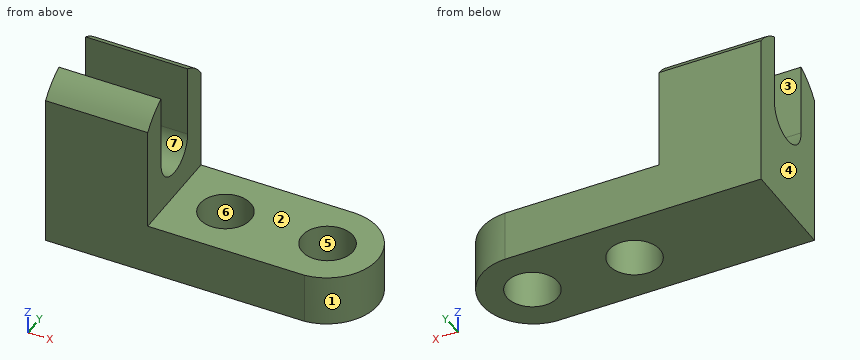
from build123d import *

# Parameters (mm, degrees)
F1_DEPTH = 25.4
F2_R     = 6.35
F3_DEPTH = 25.4
F5_DEPTH = 76.201
F7_DEPTH = 25.401
F9_DEPTH = 12.701


# Not quite as in the source:
# - ends of sketch curves that miss each other by under 0.0002 mm in the source are joined


with BuildPart() as f1:
    # F0 (on Front) → F1 (new body)
    with BuildSketch(Plane.XZ):
        Polygon((-50.8, 44.45), (-76.2, 44.45), (-76.2, 0), (0, 0), (0, 12.7), (-50.8, 12.7), align=None)
    extrude(amount=F1_DEPTH)

    # F2 (on face) → F3 (cut)
    with BuildSketch(Plane.XY.offset(12.7)):
        with Locations((-38.1, -12.7)):
            Circle(F2_R)
        with Locations((-12.7, -12.7)):
            Circle(F2_R)
    extrude(amount=-F3_DEPTH, mode=Mode.SUBTRACT)

    # F4 (on Right) → F5 (cut, through all)
    with BuildSketch(Plane.YZ):
        with BuildLine():
            ThreePointArc((-19.05, 25.4), (-12.7, 19.05), (-6.35, 25.4))
            ThreePointArc((-6.35, 25.4), (-12.7, 31.75), (-19.05, 25.4))
        make_face()
        with BuildLine():
            ThreePointArc((-19.05, 25.4), (-12.7, 31.75), (-6.35, 25.4))
            Line((-6.35, 25.4), (-6.3499049408, 44.4847454087))
            Line((-6.3499049408, 44.4847454087), (-19.05, 44.5389002562))
            Line((-19.05, 44.5389002562), (-19.05, 25.4))
        make_face()
    extrude(amount=-F5_DEPTH, mode=Mode.SUBTRACT)

    # F6 (on face) → F7 (cut, through all)
    with BuildSketch(Plane.YZ.offset(-50.8)):
        with BuildLine():
            ThreePointArc((-25.4, 38.4937003255), (-22.5556194367, 41.4256632835), (-19.05, 43.5226945042))
            Line((-19.05, 43.5226945042), (-19.05, 44.45))
            Line((-19.05, 44.45), (-25.4, 44.45))
            Line((-25.4, 44.45), (-25.4, 38.4937003255))
        make_face()
        with BuildLine():
            ThreePointArc((-6.3499103, 43.4087842374), (-2.8217014128, 41.1990275697), (0, 38.1380990148))
            Line((0, 38.1380990148), (0, 44.45))
            Line((0, 44.45), (-6.3499051138, 44.45))
            Line((-6.3499051138, 44.45), (-6.3499103, 43.4087842374))
        make_face()
    extrude(amount=-F7_DEPTH, mode=Mode.SUBTRACT)

    # F8 (on face) → F9 (cut, through all)
    with BuildSketch(Plane.XY.offset(12.7)):
        with BuildLine():
            ThreePointArc((-12.5391965152, 0), (-0.172750427, -12.3617250524), (-11.8236998096, -25.4))
            Line((-11.8236998096, -25.4), (0, -25.4))
            Line((0, -25.4), (0, 0))
            Line((0, 0), (-12.5391965152, 0))
        make_face()
    extrude(amount=-F9_DEPTH, mode=Mode.SUBTRACT)


solid = f1.part
Model file for the job. Use its own axes, mm. Face numbers are marked on the shaded views. A direction names the side the tool comes from. Give positions to 0.01 mm unless a question says otherwise; leave off trailing zeros. Order: outer loops, then holes, each group sorted by start corner. A loop starts at its lowest first (then second) coordinate and runs counter-clockwise, first axis right, second up. Notation, with made-up numbers: (58, 83.25) - (68, 83.25) arc R22 cw to (68, 96.25) - close; hole circle Ø5 at (-31.75, 44.25). An arc over 180 degrees is marked (long way). One line per item, written item: value.
Item 1: Tool access for the marked faces 1, 2 and 3: list every direction of +Z, -Z, +X, -X, +Y, -Y with a clear straight run to the whole face (end or side of a thin tool).
Response values:
face 1: +Z, -Z, +X
face 2: +Z, +X, +Y, -Y
face 3: +Z, +X, -X
Item 2: Slice it at D-D (x = -56). List the corners of the cut face in (y, z).
Response values:
outline: (-25.4, 0) - (0, 0) - (0, 38.14) arc R15.67 ccw to (-6.35, 43.41) - (-6.35, 25.4) arc R6.35 cw to (-19.05, 25.4) - (-19.05, 43.52) arc R15.67 ccw to (-25.4, 38.49) - close
Item 3: Slice it at B-B (y = -12.7). List the corners of the cut face in (x, z).
Response values:
outline: (-76.2, 0) - (-44.45, 0) - (-44.45, 12.7) - (-50.8, 12.7) - (-50.8, 19.05) - (-76.2, 19.05) - close; (-31.75, 0) - (-19.05, 0) - (-19.05, 12.7) - (-31.75, 12.7) - close; (-6.35, 0) - (-0.17, 0) - (-0.17, 12.7) - (-6.35, 12.7) - close
Item 4: Slice it at C-C (x = -38.1). List the corners of the cut face in (y, z).
Response values:
outline: (-25.4, 0) - (-19.05, 0) - (-19.05, 12.7) - (-25.4, 12.7) - close; (-6.35, 0) - (0, 0) - (0, 12.7) - (-6.35, 12.7) - close
Item 5: Slice it at A-A (z = 27). List the corners of the cut face in (x, y).
Response values:
outline: (-76.2, -25.4) - (-50.8, -25.4) - (-50.8, -19.05) - (-76.2, -19.05) - close; (-76.2, -6.35) - (-50.8, -6.35) - (-50.8, 0) - (-76.2, 0) - close
Item 6: Pin check, flat tips, straight feed: pin 1 Ø5 at (x, y) = (-16.5, -16.5) entering from +Z; pin 2 Ø12.5 at (y, z) = (-14, 27) entering from +X. Stop position of each tip, or through.
Response values:
pin 1: z = 12.7
pin 2: x = -50.8
Item 7: Wall check: line 1 (Y direction, x = -12.7, z = 8.75); line 2 (X direction, y = -7.25, z = 8.5). Give the ranges that are in metal, low to high.
Response values:
line 1: -25.4 to -19.05, -6.35 to 0
line 2: -76.2 to -41.36, -34.84 to -15.96, -9.44 to -1.4
Item 8: Two-plate mould, pull along X, no slides. Class the marked faces 4, 5, 6 and 7: released by +X, released by -X, zero draft, split by the parting line, or undercut.
Response values:
face 4: released by -X
face 5: undercut
face 6: undercut
face 7: zero draft
